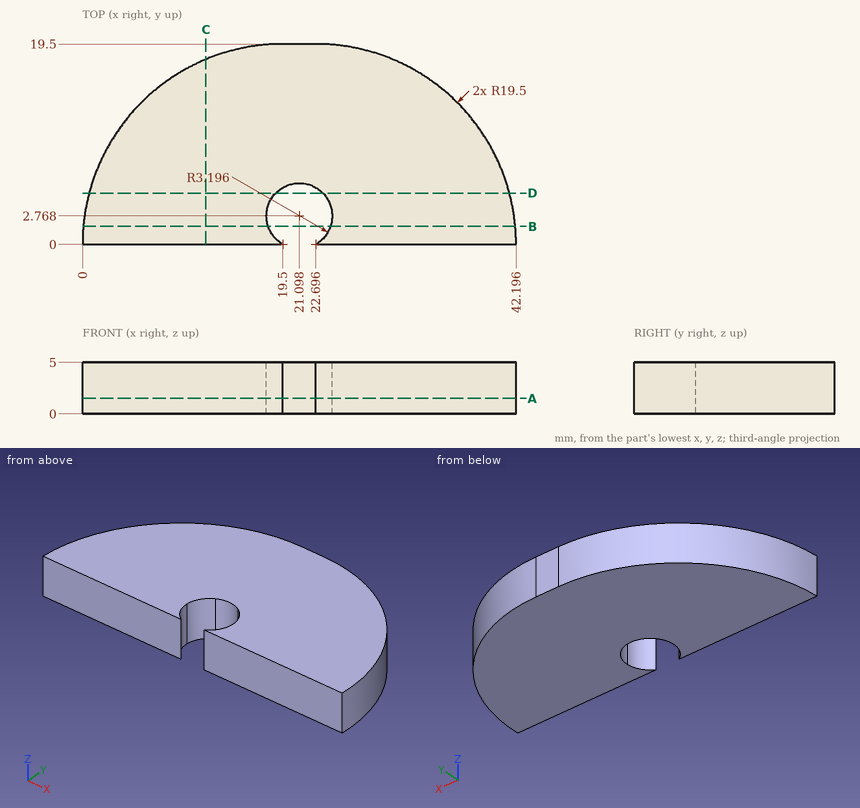
Part print with two shaded views. Sizes in mm from the minimum x, y, z corner. Coordinates: 2 decimals unless noted, no trailing zeros. Write each loop counter-clockwise with the first axis right and the second up, starting at its lowest first coordinate (ties: lowest second). Pieces come first, ordered by that corner, then holes.
1. Drop flat-ended pins along their axis: pin 1 (2 mm diameter, centred on y = 6, z = 1.5, fed in from +X); pin 2 (2 mm diameter, centred on y = 4, z = 2.5, fed in from -X). Give the stop position or say it passes through.
Answer block:
pin 1: stops at x = 41.54
pin 2: stops at x = 0.23
2. Band-saw the part on B-B, the plane y = 1.75. Give the cut face in (x, z), and give its area (3 significant figures).
Answer block:
outline: (0.08, 0) - (18.07, 0) - (18.07, 5) - (0.08, 5) - close; (24.13, 0) - (42.12, 0) - (42.12, 5) - (24.13, 5) - close
area: 180 mm2
3. Band-saw the part on C-C, the plane x = 12. Give the cut face in (y, z).
Answer block:
outline: (0, 0) - (18, 0) - (18, 5) - (0, 5) - close
4. Band-saw the part on A-A, the plane z = 1.5. Give the cut face in (x, y) (1 decimal).
Answer block:
outline: (0, 0) - (19.5, 0) arc R3.2 cw (long way) to (22.7, 0) - (42.2, 0) arc R19.5 ccw to (22.7, 19.5) - (19.5, 19.5) arc R19.5 ccw to start
5. Band-saw the part on D-D, the plane y = 5. Give the cut face in (x, z) (1 decimal), and give its area (3 significant figures).
Answer block:
outline: (0.7, 0) - (18.8, 0) - (18.8, 5) - (0.7, 5) - close; (23.4, 0) - (41.5, 0) - (41.5, 5) - (23.4, 5) - close
area: 182 mm2
6. Drill centre lines: probe 1 along X at (y, z) = (1.5, 2.6) (1 decimal); probe 2 along X at (y, z) = (2.75, 3.05) (1 decimal); probe 3 along Y at (x, z) = (23.5, 1.95) (1 decimal). Where is each one in solid material? Low to high.
Answer block:
probe 1: x = 0.1 to 18.2, 24 to 42.1
probe 2: x = 0.2 to 17.9, 24.3 to 42
probe 3: y = 0 to 0.7, 4.9 to 19.5
